Verification items for the finished model (mm, model axes). A direction names the side the tool comes from. Round coordinates to 2 decimals unless told otherwise and drop trailing zeros. Order: outer loops, then holes, each group sorted by start corner. A loop starts at its lowest first (then second) coordinate and runs counter-clockwise, first axis right, second up. Notation, with made-up numbers: (-2, 81) -> (51, 81) arc R33 ccw to (51, 109) -> close; hole circle Ø1 at (57, -36.75). An arc over 180 degrees is marked (long way). Put each result on its own line as item: value.
```python
from build123d import *

# Parameters (mm, degrees)
F0_R     = 6.35
F1_DEPTH = 63.5
F2_R     = 6.35
F3_R     = 3.175
F4_DEPTH = 6.35


with BuildPart() as f1:
    # F0 (on Front) → F1 (new body)
    with BuildSketch(Plane.XZ):
        Circle(F0_R)
    extrude(amount=F1_DEPTH)

    # F2
    f2_edges = [f1.edges().sort_by_distance(p)[0] for p in [
        (-6.35, -63.5, 0),
        (-6.35, 0, 0),
    ]]
    fillet(f2_edges, radius=F2_R)

    # F3 (on Front) → F4 (join, symmetric)
    with BuildSketch(Plane.XZ):
        Circle(F3_R)
    extrude(amount=F4_DEPTH, both=True)


solid = f1.part
```
Item 1: Sectioned sample at B-B, the plane z = 0. Record the boundary of the cut face in (x, y) (3 decimals), then the cut area to 3 significant figures.
Geometry check:
outline: (-6.35, -57.15) arc R6.35 ccw to (6.35, -57.15) -> (6.35, -6.35) arc R6.35 ccw to (3.175, -0.851) -> (3.175, 6.35) -> (-3.175, 6.35) -> (-3.175, -0.851) arc R6.35 ccw to (-6.35, -6.35) -> close
area: 814 mm2
Item 2: Sectioned sample at A-A, the plane x = 0. Record the boundary of the cut face in (y, z) (3 decimals), then the cut area to 3 significant figures.
Geometry check:
outline: (-57.15, -6.35) -> (-6.35, -6.35) arc R6.35 ccw to (-0.851, -3.175) -> (6.35, -3.175) -> (6.35, 3.175) -> (-0.851, 3.175) arc R6.35 ccw to (-6.35, 6.35) -> (-57.15, 6.35) arc R6.35 ccw to start
area: 814 mm2
Item 3: Depth check by flat-ended pin: pin 1 Ø4 at (x, z) = (-0.5, 4.5) entering from -Y; pin 2 Ø1 at (x, z) = (-2, 3.5) entering from -Y; pin 3 Ø6 at (y, z) = (-34, 0.5) entering from +X; pin 4 Ø1.5 at (y, z) = (-53, 3) entering from -X. Enter the tip coordinate at first touch or a pass-through.
Geometry check:
pin 1: y = -62.98
pin 2: y = -62.43
pin 3: x = 6.35
pin 4: x = -5.94
Item 4: Sectioned sample at C-C, the plane y = -49. Record the boundary of the cut face in (x, z), then the cut area to 3 significant figures.
Geometry check:
outline: circle Ø12.7 at (0, 0)
area: 127 mm2
Item 5: Material ranges on line 1 along X through (y, z) = (-14, 5.5); line 2 along Y through (x, z) = (-4.75, -3); line 3 along X through (y, z) = (-6, 0), recorded low to high.
Geometry check:
line 1: -3.17 to 3.17
line 2: -60.11 to -3.39
line 3: -6.34 to 6.34
Item 6: Tool access check on faces 1 (the face through (-2.52, 2.7, -1.93)), 2 (the face through (0, 6.35, 0)). Record the directions out of +Z, -Z, +X, -X, +Y, -Y that give a thin tool (end or side, any length) a straight path to the whole face; none if there is none.
Geometry check:
face 1: +Y
face 2: +Z, -Z, +X, -X, +Y
